```python
from build123d import *

# Parameters (mm, degrees)
SKETCH1_R           = 1.7
BOSS_EXTRUDE1_DEPTH = 4.87
CHAMFER1_SIZE       = 1.8
FILLET1_R           = 0.5


with BuildPart() as part:
    # Sketch1 → Boss-Extrude1 (new body)
    with BuildSketch(Plane.XY):
        with BuildLine():
            Line((-20, 0), (0, 0))
            Line((0, 0), (0, -14.062746067))
            ThreePointArc((0, -14.062746067), (-10.862024084, -10.145344108), (-20, -17.204168477))
            Line((-20, -17.204168477), (-20, 0))
        make_face()
        with Locations((-15, -8.5)):
            Circle(SKETCH1_R, mode=Mode.SUBTRACT)
        with Locations((-5, -6.5)):
            Circle(SKETCH1_R, mode=Mode.SUBTRACT)
    extrude(amount=BOSS_EXTRUDE1_DEPTH)

    # Chamfer1
    chamfer1_edges = [part.edges().sort_by_distance(p)[0] for p in [
        (-20, 0, 2.435),
        (0, 0, 2.435),
    ]]
    chamfer(chamfer1_edges, length=CHAMFER1_SIZE)

    # Fillet1
    fillet1_edges = [part.edges().sort_by_distance(p)[0] for p in [
        (0, -1.8, 2.435),
        (-20, -1.8, 2.435),
        (0, -14.062746067, 2.435),
        (-20, -17.204168477, 2.435),
    ]]
    fillet(fillet1_edges, radius=FILLET1_R)


solid = part.part
```
The listing builds one solid part. Answer for the finished solid, in the listing's coordinates (mm). Round coordinates to 2 decimals unless told otherwise and drop trailing zeros. Loops run counter-clockwise (first coordinate to the right, second up) from the corner with the lowest first, then second, coordinate; pieces in that order, holes last. Notation, with made-up numbers: (-5.75, 25.5) - (48.25, 25.5) arc R19 ccw to (48.25, 45.5) - close; hole circle Ø5 at (45.25, 58.25). An arc over 180 degrees is marked (long way). Return JSON: item names as keys, results as strings. Group by question number.
1. The part is cut by section B-B on x = -15. Determine the outline of the cut face in (y, z), then the cut area to 3 significant figures.
2. The mould has two halves that part along X. Classify faces 1 (the flat face through (-10, -6, 4.87)), 2 (the cylindrical face through (-0.29, -13.29, 2.47)), 3 (the cylindrical face through (-10.348, -10.076, 2.401)), 4 (the flat face through (-19, -0.8, 2.4)): pulls with the +X half, pulls with the -X half, needs draft (parallel to the pull), parting line crosses it, or undercut.
3. This flat-tipped pin is pushed along its axis until it touches: P1, Ø2, axis at x = -13.5, y = -9.5, coming from the -Z side. Where does it stop, or does it pass through?
4. The part is cut by section C-C on z = 0.7. Determine the outline of the cut face in (x, y).
5. The part is cut by section A-A on y = -8.5. Determine the outline of the cut face in (x, z), then the cut area to 3 significant figures.
6. The part is cut by section D-D on x = -9.75. Determine the outline of the cut face in (y, z), then the cut area to 3 significant figures.
7. Consider probe 1 along Y at (x, z) = (-5, 1.3); probe 2 along X at (y, z) = (-7.5, 2.5); probe 3 along Y at (x, z) = (-14.75, 2.5). Determine where each line is inside the solid, lowest interval first.
Resolved:
{
 "1": {"outline": "(-11.61, 0) - (-10.2, 0) - (-10.2, 4.87) - (-11.61, 4.87) - close; (-6.8, 0) - (0, 0) - (0, 4.87) - (-6.8, 4.87) - close", "area": "40.0 mm²"},
 "2": {"face 1": "needs draft", "face 2": "undercut", "face 3": "undercut", "face 4": "pulls with the -X half"},
 "3": {"P1": "stops at z = 0"},
 "4": {"outline": "(-20, -15.22) arc R0.5 ccw to (-19.08, -15.49) arc R12 cw to (-0.84, -13.2) arc R0.5 ccw to (0, -12.83) - (0, -2.01) arc R0.5 ccw to (-0.15, -1.65) - (-1.8, 0) - (-18.2, 0) - (-19.85, -1.65) arc R0.5 ccw to (-20, -2.01) - close; hole circle Ø3.4 at (-15, -8.5); hole circle Ø3.4 at (-5, -6.5)"},
 "5": {"outline": "(-20, 0) - (-16.7, 0) - (-16.7, 4.87) - (-20, 4.87) - close; (-13.3, 0) - (0, 0) - (0, 4.87) - (-13.3, 4.87) - close", "area": "80.8 mm²"},
 "6": {"outline": "(-10.02, 0) - (0, 0) - (0, 4.87) - (-10.02, 4.87) - close", "area": "48.8 mm²"},
 "7": {"probe 1": "y = -10.69 to -8.2, -4.8 to 0", "probe 2": "x = -20 to -16.37, -13.63 to -6.37, -3.63 to 0", "probe 3": "y = -11.47 to -10.18, -6.82 to 0"}
}
